```python
from build123d import *

# Parameters (mm, degrees)
SKETCH1_R           = 10
SKETCH1_R_2         = 5
BOSS_EXTRUDE1_DEPTH = 10
SKETCH2_R           = 2
BOSS_EXTRUDE2_DEPTH = 5
SKETCH3_R           = 1.5
CUT_EXTRUDE1_DEPTH  = 26
FILLET1_R           = 1


with BuildPart() as part:
    # Sketch1 → Boss-Extrude1 (new body)
    with BuildSketch(Plane(origin=(0, 0, 0), x_dir=(1, 0, 0), z_dir=(0, 1, 0))):
        Circle(SKETCH1_R)
        Circle(SKETCH1_R_2, mode=Mode.SUBTRACT)
    extrude(amount=BOSS_EXTRUDE1_DEPTH)

    # Sketch2 → Boss-Extrude2 (add)
    with BuildSketch(Plane(origin=(0, 10, 0), x_dir=(1, 0, 0), z_dir=(0, 1, 0))):
        with BuildLine():
            Line((-21, -25), (21, -25))
            ThreePointArc((21, -25), (23.828427125, -23.828427125), (25, -21))
            Line((25, -21), (25, 21))
            ThreePointArc((25, 21), (23.828427125, 23.828427125), (21, 25))
            Line((21, 25), (-21, 25))
            ThreePointArc((-21, 25), (-23.828427125, 23.828427125), (-25, 21))
            Line((-25, 21), (-25, -21))
            ThreePointArc((-25, -21), (-23.828427125, -23.828427125), (-21, -25))
        make_face()
        with Locations((-20, 20)):
            Circle(SKETCH2_R, mode=Mode.SUBTRACT)
        with Locations((20, 20)):
            Circle(SKETCH2_R, mode=Mode.SUBTRACT)
        with Locations((20, -20)):
            Circle(SKETCH2_R, mode=Mode.SUBTRACT)
        with Locations((-20, -20)):
            Circle(SKETCH2_R, mode=Mode.SUBTRACT)
    extrude(amount=BOSS_EXTRUDE2_DEPTH)

    # Sketch3 → Cut-Extrude1 (cut, through all)
    with BuildSketch(Plane.XY):
        with Locations((0, 5)):
            Circle(SKETCH3_R)
    extrude(amount=CUT_EXTRUDE1_DEPTH, mode=Mode.SUBTRACT)

    # Fillet1
    fillet1_edges = [part.edges().sort_by_distance(p)[0] for p in [
        (0, 15, 25),
        (23.828427125, 15, 23.828427125),
        (25, 15, 0),
        (23.828427125, 15, -23.828427125),
        (0, 15, -25),
        (-23.828427125, 15, -23.828427125),
        (-25, 15, 0),
        (-23.828427125, 10, 23.828427125),
        (0, 10, 25),
        (23.828427125, 10, 23.828427125),
        (25, 10, 0),
        (23.828427125, 10, -23.828427125),
        (0, 10, -25),
        (-23.828427125, 10, -23.828427125),
        (-25, 10, 0),
        (-23.828427125, 15, 23.828427125),
    ]]
    fillet(fillet1_edges, radius=FILLET1_R)


solid = part.part
```
Check sheet for the modelled part. Datum: model origin and axes. Units: mm. A direction names the side the tool comes from. Coordinates: 2 decimals unless noted, no trailing zeros. Write each loop counter-clockwise with the first axis right and the second up, starting at its lowest first coordinate (ties: lowest second). Pieces come first, ordered by that corner, then holes. Notation, with made-up numbers: M 27,25.25 L 80,25.25 A24 cw 80,52.25 Z; hole C -9,-37.75 d4. An arc over 180 degrees is marked long. Write item = value, one per line. Start each with the question number.
1. Thickness scan on probe 1 along X at (y, z) = (11.8, -20); probe 2 along X at (y, z) = (13, 18.5). Record the ranges inside material, lowest first.
2. Sectioned sample at A-A (x = 0). Record the cut outline in (y, z), then the cut area to 3 significant figures.
3. Sectioned sample at C-C (x = 20). Record the cut outline in (y, z).
4. Sectioned sample at B-B (y = 13.25). Record the cut outline in (x, z).
5. Sectioned sample at D-D (z = 20). Record the cut outline in (x, y), then the cut area to 3 significant figures.
6. Tool access check on faces 1 (the cylindrical face through (3, 5, -4)), 2 (the cylindrical face through (-1.5, 5.07, 7.35)), 3 (the cylindrical face through (-23.859, 12.479, 23.797)). Record the directions out of +Z, -Z, +X, -X, +Y, -Y that give a thin tool (end or side, any length) a straight path to the whole face; none if there is none.
7. Go/stop test with flat-tipped pins: pin 1 (2 mm diameter, centred on y = 8.5, z = -0.5, fed in from -X); pin 2 (5 mm diameter, centred on x = -8.5, y = 5, fed in from -Z); pin 3 (1.5 mm diameter, centred on x = 10, z = 10.5, fed in from -Y); pin 4 (2.5 mm diameter, centred on x = 20, z = 20, fed in from +Y). Record where each tip stops, or that it passes through.
8. Mould release check, pull along X, two halves, no side actions. Record for faces 4 (the cylindrical face through (23.797, 12.479, 23.859)), 5 (the flat face through (0, 15, 0)), 6 (the cylindrical face through (20, 12, -22)): pulls with the +X half, pulls with the -X half, needs draft (parallel to the pull), parting line crosses it, or undercut.
The answers:
q1.probe_1 = -25 to -22, -18 to 18, 22 to 25
q1.probe_2 = -25 to -21.32, -18.68 to 18.68, 21.32 to 25
q2.outline = M 0,-10 L 10,-10 L 10,-24 A1 ccw 11,-25 L 14,-25 A1 ccw 15,-24 L 15,24 A1 ccw 14,25 L 11,25 A1 ccw 10,24 L 10,10 L 6.5,10 L 6.5,5 L 10,5 L 10,-5 L 0,-5 Z; M 0,5 L 3.5,5 L 3.5,10 L 0,10 Z
q2.area = 334 mm²
q3.outline = M 10,-24 A1 ccw 11,-25 L 14,-25 A1 ccw 15,-24 L 15,-22 L 10,-22 Z; M 10,-18 L 15,-18 L 15,18 L 10,18 Z; M 10,22 L 15,22 L 15,24 A1 ccw 14,25 L 11,25 A1 ccw 10,24 Z
q4.outline = M -25,-21 A4 ccw -21,-25 L 21,-25 A4 ccw 25,-21 L 25,21 A4 ccw 21,25 L -21,25 A4 ccw -25,21 Z; hole C -20,-20 d4; hole C -20,20 d4; hole C 20,-20 d4; hole C 20,20 d4
q5.outline = M -25,11 A1 ccw -24,10 L -22,10 L -22,15 L -24,15 A1 ccw -25,14 Z; M -18,10 L 18,10 L 18,15 L -18,15 Z; M 22,10 L 24,10 A1 ccw 25,11 L 25,14 A1 ccw 24,15 L 22,15 Z
q5.area = 209 mm²
q6.face_1 = -Y
q6.face_2 = +Z
q6.face_3 = +Z, -X, +Y, -Y
q7.pin_1 = -10
q7.pin_2 = -8
q7.pin_3 = 10
q7.pin_4 = through
q8.face_4 = pulls with the +X half
q8.face_5 = needs draft
q8.face_6 = undercut
